```python
from build123d import *

# Parameters (mm, degrees)
SKETCH1_W               = 50
SKETCH1_H               = 50
BOSS_EXTRUDE1_DEPTH     = 50
BOSS_EXTRUDE2_DEPTH     = 50
SKETCH4_W               = 18.75
SKETCH4_H               = 70.710678119
CUT_EXTRUDE2_DEPTH      = 100
CUT_EXTRUDE2_DEPTH_BACK = 100
SKETCH5_R               = 18.75
SKETCH6_W               = 50
SKETCH6_H               = 50
BOSS_EXTRUDE3_DEPTH     = 5
SKETCH7_W               = 18.75
SKETCH7_H               = 70.710678119
SKETCH9_R               = 18.867934004
BOSS_EXTRUDE6_DEPTH     = 20
SKETCH10_W              = 50
SKETCH10_H              = 65.146880585
CUT_EXTRUDE3_DEPTH      = 40
CUT_EXTRUDE4_START      = -70
SKETCH11_R              = 18.75
CUT_EXTRUDE4_DEPTH      = 70
SKETCH12_W              = 50
SKETCH12_H              = 46.047099175
BOSS_EXTRUDE7_DEPTH     = 5
SKETCH13_R              = 2.4
SKETCH13_R_2            = 2.5
CUT_EXTRUDE5_DEPTH      = 5


with BuildPart() as part:
    # Sketch1 → Boss-Extrude1 (new body)
    with BuildSketch(Plane.XY):
        with Locations((-25, 25)):
            Rectangle(SKETCH1_W, SKETCH1_H)
    extrude(amount=BOSS_EXTRUDE1_DEPTH)

    # Sketch2 → Boss-Extrude2 (add)
    with BuildSketch(Plane.XY.offset(50)):
        Polygon((0, 50), (-50, 50), (-50, 100), align=None)
    extrude(amount=-BOSS_EXTRUDE2_DEPTH)

    # Sketch4 → Revolve1 (revolve)
    with BuildSketch(Plane(origin=(25, 25, 0), x_dir=(0, 0, -1), z_dir=(0.7071067811865477, 0.7071067811865475, 0))):
        with Locations((-34.375, 70.710678118)):
            Rectangle(SKETCH4_W, SKETCH4_H)
    revolve(axis=Axis((-50, 100, 25), (0.7071067811865475, -0.7071067811865477, 0)))

    # Sketch5 → Cut-Extrude2 (cut, two sides: drawn at the far end of the back side and taken through both)
    with BuildSketch(Plane(origin=(-25, 25, 0), x_dir=(0, 0, -1), z_dir=(0.7071067811865477, -0.7071067811865475, 0)).offset(-CUT_EXTRUDE2_DEPTH_BACK)):
        with Locations((-25, 35.355339059)):
            Circle(SKETCH5_R)
    extrude(amount=CUT_EXTRUDE2_DEPTH + CUT_EXTRUDE2_DEPTH_BACK, mode=Mode.SUBTRACT)

    # Sketch6 → Boss-Extrude3 (add)
    with BuildSketch(Plane.XZ):
        Polygon((-70, 0), (-70, -20), (-50, -20), (20, -20), (20, 50), (20, 70), (0, 70), (-70, 70), align=None)
        with Locations((-25, 25)):
            Rectangle(SKETCH6_W, SKETCH6_H, mode=Mode.SUBTRACT)
    extrude(amount=-BOSS_EXTRUDE3_DEPTH)

    # Sketch7 → Revolve2 (revolve)
    with BuildSketch(Plane(origin=(25, 25, 0), x_dir=(0, 0, -1), z_dir=(0.7071067811865477, 0.7071067811865475, 0))):
        with Locations((-34.375, 70.710678118)):
            Rectangle(SKETCH7_W, SKETCH7_H)
    revolve(axis=Axis((0, 50, 25), (-0.7071067811865475, 0.7071067811865477, 0)))

    # Sketch9 → Boss-Extrude6 (add)
    with BuildSketch(Plane(origin=(-25, 25, 0), x_dir=(0, 0, -1), z_dir=(0.7071067811865477, -0.7071067811865475, 0))):
        with Locations(Location((-25.10968595, 35.312009835, 0), (0, 0, 179.868423122))):
            Circle(SKETCH9_R)
    extrude(amount=BOSS_EXTRUDE6_DEPTH)

    # Sketch10 → Cut-Extrude3 (cut)
    with BuildSketch(Plane(origin=(0, 0, 0), x_dir=(0, 0, -1), z_dir=(1, 0, 0))):
        with Locations((-25, 49.118259987)):
            Rectangle(SKETCH10_W, SKETCH10_H)
    extrude(amount=CUT_EXTRUDE3_DEPTH, mode=Mode.SUBTRACT)

    # Sketch11 → Cut-Extrude4 (cut)
    with BuildSketch(Plane(origin=(-75, 75, 0), x_dir=(0, 0, 1), z_dir=(-0.7071067811865477, 0.7071067811865475, 0)).offset(CUT_EXTRUDE4_START)):
        with Locations((25, 35.355339059)):
            Circle(SKETCH11_R)
    extrude(amount=CUT_EXTRUDE4_DEPTH, mode=Mode.SUBTRACT)

    # Sketch12 → Boss-Extrude7 (add)
    with BuildSketch(Plane(origin=(0, 0, 0), x_dir=(0, 0, -1), z_dir=(1, 0, 0))):
        with Locations((-25, 28.023549588)):
            Rectangle(SKETCH12_W, SKETCH12_H)
    extrude(amount=BOSS_EXTRUDE7_DEPTH)

    # Sketch13 → Cut-Extrude5 (cut)
    with BuildSketch(Plane(origin=(0, 5, 0), x_dir=(1, 0, 0), z_dir=(0, 1, 0))):
        with Locations(Location((5, 6, 0), (0, 0, 270))):
            Circle(SKETCH13_R)
        with Locations(Location((5, -54, 0), (0, 0, 270))):
            Circle(SKETCH13_R)
        with Locations(Location((-55, 6, 0), (0, 0, 270))):
            Circle(SKETCH13_R_2)
        with Locations(Location((-55, -54, 0), (0, 0, 270))):
            Circle(SKETCH13_R_2)
    extrude(amount=-CUT_EXTRUDE5_DEPTH, mode=Mode.SUBTRACT)


solid = part.part
```
Could you check a few things on this model? Use its own coordinates, in mm. A direction names the side the tool comes from. Give positions to 0.01 mm unless a question says otherwise; leave off trailing zeros. Order: outer loops, then holes, each group sorted by start corner. A loop starts at its lowest first (then second) coordinate and runs counter-clockwise, first axis right, second up.
Q1. Suppose I cut it at D-D, the plane z = 18. Write out the boundary of the cut face in (x, y), and give its area (3 significant figures).
Q2. We'd pull the mould along Z, two halves only. Please class faces 1 (the flat face through (-24, 2, 70)), 2 (the flat face through (-26, 0, 26)), 3 (the cylindrical face through (7.38, 2.54, 53.69)): +Z half, -Z half, draft (parallel to the pull), parting line (faces both ways), or undercut.
Q3. I'm going to push flat-ended pins straight in: P1, Ø10, axis at x = 0.5, z = 4.5, coming from the +Y side; P2, Ø1.5, axis at x = -37.5, y = 43, coming from the +Z side; P3, Ø15, axis at y = 51, z = 22.5, coming from the -X side; P4, Ø6, axis at x = -7.5, z = 53.5, coming from the -Y side. Where does each tip first touch, or does it pass through?
Q4. For faces 4 (the flat face through (-29, 41, 50)), 5 (the cylindrical face through (-32.66, 56.15, 24.59)), 6 (the flat face through (2, 51.047, 25)), which set-ups out of +Z, -Z, +X, -X, +Y, -Y let a thin tool reach every point of the face, with its end or its side?
Q5. Suppose I cut it at C-C, the plane y = 31. Write out the boundary of the cut face in (x, z).
Q6. If I drill on line 1 along X through (y, z) = (2, 54); line 2 along Y through (x, z) = (15, -1); line 3 along X through (y, z) = (40, 30.5), over which ranges is the centre line in solid material (lowest first)?
Q7. Suppose I cut it at B-B, the plane x = -55. Write out the boundary of the cut face in (y, z).
Q8. Suppose I cut it at A-A, the plane z = 54. Write out the boundary of the cut face in (x, y), and give its area (3 significant figures).
Solution:
1. outline: (-70, 0) - (20, 0) - (20, 5) - (5, 5) - (5, 51.05) - (0, 51.05) - (0, 51.01) - (-12.8, 38.2) - (-50, 75.4) - (-50, 5) - (-70, 5) - close
1. area: 3,110 mm2
2. face 1: +Z half
2. face 2: draft
2. face 3: undercut
3. P1: stops at y = 54.5
3. P2: stops at z = 50
3. P3: stops at x = -50
3. P4: stops at y = 0
4. face 4: +Z, +X, -X, +Y
4. face 5: +Y
4. face 6: +Z, -Z, +X, +Y
5. outline: (-50, 0) - (5, 0) - (5, 50) - (-50, 50) - close
6. line 1: x = -70 to -57.5, -52.5 to 2.6, 7.4 to 20
6. line 2: y = 0 to 5
6. line 3: x = -50 to -15.35, -11.01 to 5
7. outline: (0, -20) - (5, -20) - (5, -8.5) - (0, -8.5) - close; (0, -3.5) - (5, -3.5) - (5, 51.5) - (0, 51.5) - close; (0, 56.5) - (5, 56.5) - (5, 70) - (0, 70) - close
8. outline: (-70, 0) - (-57.5, 0) - (-57.5, 5) - (-70, 5) - close; (-52.5, 0) - (2.6, 0) - (2.6, 5) - (-52.5, 5) - close; (7.4, 0) - (20, 0) - (20, 5) - (7.4, 5) - close
8. area: 401 mm2
